Work out the finished part from the listing and answer in its coordinate system (mm). A direction names the side the tool comes from. Coordinates: 2 decimals unless noted, no trailing zeros. Write each loop counter-clockwise with the first axis right and the second up, starting at its lowest first coordinate (ties: lowest second). Pieces come first, ordered by that corner, then holes. Notation, with made-up numbers: M 72.25,67 L 86.25,67 A36 ccw 86.25,105 Z; hole C 43,40 d10. An arc over 180 degrees is marked long. Use CSV: the item, a comma, the result in double quotes.
Autodesk Inventor part; units mm, degrees
ref_plane "YZ Plane" through (0, 0, 0) normal (1, 0, 0) x (0, 1, 0)
ref_plane "XZ Plane" through (0, 0, 0) normal (0, 1, 0) x (-1, 0, 0)
ref_plane "XY Plane" through (0, 0, 0) normal (0, 0, 1) x (1, 0, 0)
sketch "Sketch1" plane through (0, 0, 0) normal (0, 1, 0) x (-1, 0, 0)
  circle A0 centre (0, 0) radius 4.5
  dimension "d0" = 9
extrude "Extrusion1" add sketch "Sketch1" along normal blind 6.5
sketch "Sketch2" plane through (0, 6.5, 0) normal (0, 1, 0) x (1, 0, 0)
  circle A0 centre (0, 0) radius 3.565
  dimension "d3" = 7.13
extrude "Extrusion2" add sketch "Sketch2" along normal blind 7
sketch "Sketch3" plane through (0, 13.5, 0) normal (0, 1, 0) x (1, 0, 0)
  circle A0 centre (0, 0) radius 4.5
  dimension "d6" = 9
extrude "Extrusion3" add sketch "Sketch3" along normal blind 6.5
sketch "Sketch4" plane through (0, 20, 0) normal (0, 1, 0) x (1, 0, 0)
  circle A0 centre (0, 0) radius 1.6
  dimension "d9" = 3.2
extrude "Extrusion4" cut sketch "Sketch4" against normal blind 20
sketch "Sketch5" plane through (0, 0, 0) normal (0, -1, 0) x (1, 0, 0)
  circle A0 centre (0, 0) radius 1.6
  circle A1 centre (0, 0) radius 2
  dimension "d12" = 4
extrude "Extrusion5" cut sketch "Sketch5" against normal blind 10
properties part number "coupler" material "Gold"
Item 1: Consider probe 1 along Z at (x, y) = (0, 13) (3 decimals); probe 2 along Z at (x, y) = (0, 14); probe 3 along Y at (x, z) = (3.25, 2.75). Determine where each line is inside the solid, lowest interval first.
Answer:
probe 1,"z = -3.565 to -1.6, 1.6 to 3.565"
probe 2,"z = -4.5 to -1.6, 1.6 to 4.5"
probe 3,"y = 0 to 6.5, 13.5 to 20"
Item 2: Given pin 1 (1 mm diameter, centred on x = -2.5, y = 2, fed in from +Z); pin 2 (1 mm diameter, centred on x = -1, y = 3.5, fed in from -Z); pin 3 (3.5 mm diameter, centred on x = 0, z = 0, fed in from -Y), each flat-ended and moving along its own axis, determine where each tip first touches the part or whether it passes through.
Answer:
pin 1,"stops at z = 4.03"
pin 2,"stops at z = -4.47"
pin 3,"stops at y = 10"
Item 3: The part is cut by section D-D (x = -2.75). Write down the section's boundary in (y, z), then the cut area to 3 significant figures.
Answer:
outline,"M 0,-3.56 L 6.5,-3.56 L 6.5,-2.27 L 13.5,-2.27 L 13.5,-3.56 L 20,-3.56 L 20,3.56 L 13.5,3.56 L 13.5,2.27 L 6.5,2.27 L 6.5,3.56 L 0,3.56 Z"
area,"124 mm2"
Item 4: The part is cut by section A-A (x = 0). Write down the section's boundary in (y, z) (3 decimals).
Answer:
outline,"M 0,-4.5 L 6.5,-4.5 L 6.5,-3.565 L 13.5,-3.565 L 13.5,-4.5 L 20,-4.5 L 20,-1.6 L 10,-1.6 L 10,-2 L 0,-2 Z; M 0,2 L 10,2 L 10,1.6 L 20,1.6 L 20,4.5 L 13.5,4.5 L 13.5,3.565 L 6.5,3.565 L 6.5,4.5 L 0,4.5 Z"
Item 5: For a pull along X with two mould halves and no side action, classify faces 3 (the face through (0, 5, -2)), 4 (the face through (0.59, 3.2, -4.46)), 5 (the face through (0, 20, 2)) as released by +X, released by -X, zero draft, split by the parting line, or undercut.
Answer:
face 3,"undercut"
face 4,"split by the parting line"
face 5,"zero draft"
Item 6: The part is cut by section B-B (z = 0). Write down the section's boundary in (x, y) (3 decimals), then the cut area to 3 significant figures.
Answer:
outline,"M -4.5,0 L -2,0 L -2,10 L -1.6,10 L -1.6,20 L -4.5,20 L -4.5,13.5 L -3.565,13.5 L -3.565,6.5 L -4.5,6.5 Z; M 1.6,10 L 2,10 L 2,0 L 4.5,0 L 4.5,6.5 L 3.565,6.5 L 3.565,13.5 L 4.5,13.5 L 4.5,20 L 1.6,20 Z"
area,"94.9 mm2"
Item 7: A tool of negligible diameter and unlimited length cuts with its end or side. For faces 1 (the face through (-1.27, 15.07, 0.97)), 2 (the face through (3.4, 9.95, 1.07)), from which of +Z, -Z, +X, -X, +Y, -Y can it reach the whole face along a straight path? Write none if from no direction.
Answer:
face 1,"+Y, -Y"
face 2,"none"
Item 8: The part is cut by section C-C (y = 12). Write down the section's boundary in (x, z) (3 decimals), then the cut area to 3 significant figures.
Answer:
outline,"C 0,0 d7.13; hole C 0,0 d3.2"
area,"31.9 mm2"
